Can you work these out from the model? Positions are in its coordinate system, mm. Face numbers are marked on the shaded views. Give positions to 0.01 mm unless a question says otherwise; leave off trailing zeros. Loops run counter-clockwise (first coordinate to the right, second up) from the corner with the lowest first, then second, coordinate; pieces in that order, holes last.
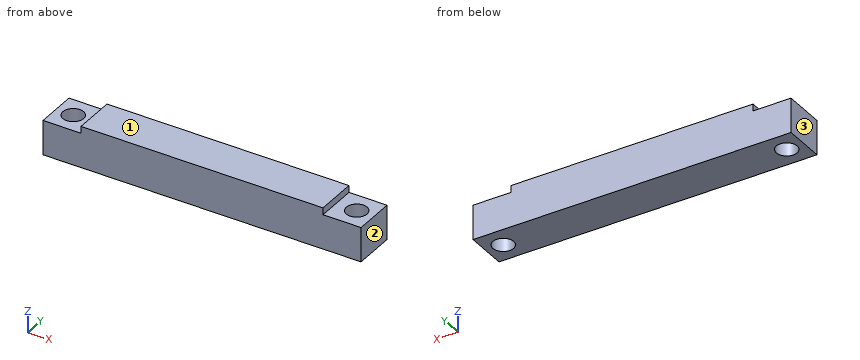
from build123d import *

# Parameters (mm, degrees)
SKETCH1_W           = 5.5
SKETCH1_H           = 6
SKETCH1_R           = 1.5
SKETCH1_W_2         = 35
BOSS_EXTRUDE1_DEPTH = 5
SKETCH1_3_W         = 35
SKETCH1_3_H         = 6
BOSS_EXTRUDE2_DEPTH = 6


with BuildPart() as part:
    # Sketch1 → Boss-Extrude1 (new body)
    # profile 1 of 3: a face of its own
    with BuildSketch(Plane.XY):
        with Locations((-20.25, 0)):
            Rectangle(SKETCH1_W, SKETCH1_H)
        with Locations((-20.5, 0)):
            Circle(SKETCH1_R, mode=Mode.SUBTRACT)
    # profile 2 of 3: a face of its own
    with BuildSketch(Plane.XY):
        with Locations((20.25, 0)):
            Rectangle(SKETCH1_W, SKETCH1_H)
        with Locations((20.5, 0)):
            Circle(SKETCH1_R, mode=Mode.SUBTRACT)
    # profile 3 of 3: a face of its own
    with BuildSketch(Plane.XY):
        Rectangle(SKETCH1_W_2, SKETCH1_H)
    extrude(amount=BOSS_EXTRUDE1_DEPTH)

    # Sketch1_3 → Boss-Extrude2 (add)
    with BuildSketch(Plane.XY):
        Rectangle(SKETCH1_3_W, SKETCH1_3_H)
    extrude(amount=BOSS_EXTRUDE2_DEPTH)


solid = part.part
(1) Thinking about a two-plate mould opening in X: for the marked faces 1, 2 and 3, which applies, pulls with the +X half, pulls with the -X half, needs draft (parallel to the pull), parting line crosses it, or undercut?
Returned:
face 1: needs draft
face 2: pulls with the +X half
face 3: pulls with the -X half
(2) Please list where these lines run through material, in increasing order: probe 1 along X at (y, z) = (-0.1, 3.2); probe 2 along X at (y, z) = (-0.95, 4.15); probe 3 along Y at (x, z) = (-20.5, 1.9).
Returned:
probe 1: x = -23 to -22, -19 to 19, 22 to 23
probe 2: x = -23 to -21.66, -19.34 to 19.34, 21.66 to 23
probe 3: y = -3 to -1.5, 1.5 to 3
(3) Suppose I cut it at B-B on y = 0. List the corners of the cut face in (x, z) for me.
Returned:
outline: (-23, 0) - (-22, 0) - (-22, 5) - (-23, 5) - close; (-19, 0) - (19, 0) - (19, 5) - (17.5, 5) - (17.5, 6) - (-17.5, 6) - (-17.5, 5) - (-19, 5) - close; (22, 0) - (23, 0) - (23, 5) - (22, 5) - close
(4) Will these pins go through, and if not, where does the flat tip stop? P1, Ø1.6, axis at x = 19, y = -1.5, coming from the +Z side; P2, Ø2.5, axis at x = 20.5, y = 0, coming from the -Z side.
Returned:
P1: stops at z = 5
P2: passes through
(5) Suppose I cut it at A-A on x = -20.5. List the corners of the cut face in (y, z) for me.
Returned:
outline: (-3, 0) - (-1.5, 0) - (-1.5, 5) - (-3, 5) - close; (1.5, 0) - (3, 0) - (3, 5) - (1.5, 5) - close
(6) Suppose I cut it at D-D on y = -2.15. List the corners of the cut face in (x, z) for me, plus the area to 3 significant figures.
Returned:
outline: (-23, 0) - (23, 0) - (23, 5) - (17.5, 5) - (17.5, 6) - (-17.5, 6) - (-17.5, 5) - (-23, 5) - close
area: 265 mm2
(7) Suppose I cut it at C-C on z = 3.1. List the corners of the cut face in (x, y) for me, plus the area to 3 significant figures.
Returned:
outline: (-23, -3) - (23, -3) - (23, 3) - (-23, 3) - close; hole circle Ø3 at (-20.5, 0); hole circle Ø3 at (20.5, 0)
area: 262 mm2
